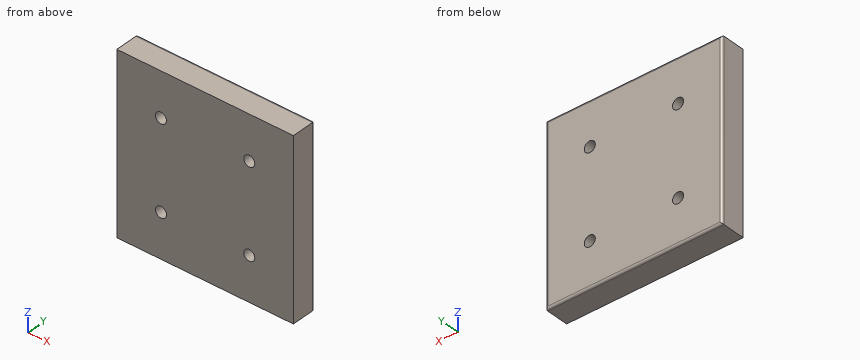
from build123d import *

# Parameters (mm, degrees)
SKETCH_1_W                  = 160
SKETCH_1_H                  = 160
EXTRUDE_1_DEPTH             = 22.5
SKETCH_2_R                  = 5
CUT_EXTRUDE_1_DEPTH         = 228.390083337
PATTERN_LINEAR_1_COUNT      = 2
PATTERN_LINEAR_1_PITCH      = 80
PATTERN_LINEAR_1_COUNT_DIR2 = 2
PATTERN_LINEAR_1_PITCH_DIR2 = 80
FILLET_2_R                  = 2


with BuildPart() as part:
    # 草图1 → 凸台-拉伸1 (new body)
    with BuildSketch(Plane(origin=(0, 0, 0), x_dir=(1, 0, 0), z_dir=(0, 1, 0))):
        with Locations((80, 80)):
            Rectangle(SKETCH_1_W, SKETCH_1_H)
    extrude(amount=EXTRUDE_1_DEPTH)

    # 草图2 → 切除-拉伸1 (cut, through all)
    with BuildSketch(Plane(origin=(0, 22.5, 0), x_dir=(1, 0, 0), z_dir=(0, 1, 0))):
        with Locations(Location((40, 120, 0), (0, 0, 270))):
            Circle(SKETCH_2_R)
    cut_extrude_1 = extrude(amount=-CUT_EXTRUDE_1_DEPTH, mode=Mode.SUBTRACT)

    # 阵列(线性)1: Cut-Extrude 1 2 × 2
    with Locations(*[(i * PATTERN_LINEAR_1_PITCH, 0, j * PATTERN_LINEAR_1_PITCH_DIR2) for i in range(PATTERN_LINEAR_1_COUNT) for j in range(PATTERN_LINEAR_1_COUNT_DIR2) if (i, j) != (0, 0)]):
        add(cut_extrude_1, mode=Mode.SUBTRACT)

    # 圆角2
    fillet_2_edges = [part.edges().sort_by_distance(p)[0] for p in [
        (160, 22.5, -80),
        (80, 22.5, -160),
        (0, 22.5, -80),
        (80, 22.5, 0),
    ]]
    fillet(fillet_2_edges, radius=FILLET_2_R)


solid = part.part
The model under review builds one solid part; all positions refer to its coordinate system, in mm. Coordinates: 2 decimals unless noted, no trailing zeros. Write each loop counter-clockwise with the first axis right and the second up, starting at its lowest first coordinate (ties: lowest second). Pieces come first, ordered by that corner, then holes. Notation, with made-up numbers: (63, 21) - (118, 21) arc R9 ccw to (118, 27) - close; hole circle Ø8 at (50, 34.5). An arc over 180 degrees is marked (long way). Answer as CSV lines item,"result".
(1) For line 1 along X through (y, z) = (15.25, -40); line 2 along Z through (x, y) = (44, 20.75); line 3 along X through (y, z) = (1.75, -122.5), list the stretches that pass through material, from the lowest coordinate up. Write a range as [from, to].
Data:
line 1,"x = [0, 35], [45, 115], [125, 160]"
line 2,"z = [-159.98, -123], [-117, -43], [-37, -0.02]"
line 3,"x = [0, 35.67], [44.33, 115.67], [124.33, 160]"
(2) We need section A-A (x = 40). Give the boundary of the cut face in (y, z).
Data:
outline,"(0, -160) - (20.5, -160) arc R2 ccw to (22.5, -158) - (22.5, -125) - (0, -125) - close; (0, -115) - (22.5, -115) - (22.5, -45) - (0, -45) - close; (0, -35) - (22.5, -35) - (22.5, -2) arc R2 ccw to (20.5, 0) - (0, 0) - close"
(3) We need section B-B (z = -40). Give the boundary of the cut face in (x, y).
Data:
outline,"(0, 0) - (35, 0) - (35, 22.5) - (2, 22.5) arc R2 ccw to (0, 20.5) - close; (45, 0) - (115, 0) - (115, 22.5) - (45, 22.5) - close; (125, 0) - (160, 0) - (160, 20.5) arc R2 ccw to (158, 22.5) - (125, 22.5) - close"
